from build123d import *

# Parameters (mm, degrees)
F0_W     = 330.2
F0_H     = 173.9225888619
F0_R     = 66.675
F1_DEPTH = 6.35


# Not quite as in the source:
# - the dataset's text gives a spline's control points without its knots; the knots are read off the source's solid


with BuildPart() as f1:
    # F0 (on Top) → F1 (new body)
    with BuildSketch(Plane.XY):
        with Locations((-132.4583572531, -73.9906652679)):
            Rectangle(F0_W, F0_H)
        with BuildLine():
            add(Edge.make_bspline(
                [(-138.9201402808, -141.3304854369), (-138.3928185407, -141.3304854369), (-137.3381750605, -141.275400301), (-135.2625215798, -140.9492902881), (-133.2552416123, -140.3064688013), (-131.3632448334, -139.3625418043), (-129.5649193209, -138.2239224731), (-127.5612000685, -136.4834555233), (-125.9244832491, -134.3798930655), (-124.862585277, -132.5093025607), (-123.9869219901, -130.5516065921), (-123.3950651292, -128.4884227829), (-123.095646983, -126.3629935264), (-123.0198869297, -124.7450926538), (-123.095646983, -123.1271917812), (-123.3950651292, -121.0017625246), (-123.9869219901, -118.9385787154), (-124.862585277, -116.9808827469), (-125.9244832491, -115.110292242), (-127.5612000685, -113.0067297843), (-129.5649193209, -111.2662628345), (-131.3632448334, -110.1276435032), (-133.2552416123, -109.1837165063), (-135.2625215798, -108.5408950195), (-137.3381750605, -108.2147850066), (-138.9201402808, -108.1321573027), (-140.5021055011, -108.2147850066), (-142.5777589818, -108.5408950195), (-144.5850389493, -109.1837165063), (-146.4770357282, -110.1276435032), (-148.2753612407, -111.2662628345), (-150.2790804931, -113.0067297843), (-151.9157973125, -115.110292242), (-152.9776952845, -116.9808827469), (-153.8533585715, -118.9385787154), (-154.4452154324, -121.0017625246), (-154.7446335786, -123.1271917812), (-154.8203936319, -124.7450926538), (-154.7446335786, -126.3629935264), (-154.4452154324, -128.4884227829), (-153.8533585715, -130.5516065921), (-152.9776952845, -132.5093025607), (-151.9157973125, -134.3798930655), (-150.2790804931, -136.4834555233), (-148.2753612407, -138.2239224731), (-146.4770357282, -139.3625418043), (-144.5850389493, -140.3064688013), (-142.5777589818, -140.9492902881), (-140.5021055011, -141.275400301), (-139.4474620209, -141.3304854369), (-138.9201402808, -141.3304854369)],
                knots=[0, 0, 0, 0, 0.015625, 0.03125, 0.0625, 0.078125, 0.09375, 0.125, 0.15625, 0.171875, 0.1875, 0.21875, 0.234375, 0.25, 0.265625, 0.28125, 0.3125, 0.328125, 0.34375, 0.375, 0.40625, 0.421875, 0.4375, 0.46875, 0.484375, 0.5, 0.515625, 0.53125, 0.5625, 0.578125, 0.59375, 0.625, 0.65625, 0.671875, 0.6875, 0.71875, 0.734375, 0.75, 0.765625, 0.78125, 0.8125, 0.828125, 0.84375, 0.875, 0.90625, 0.921875, 0.9375, 0.96875, 0.984375, 1, 1, 1, 1], degree=3))
        make_face(mode=Mode.SUBTRACT)
        with Locations((-219.2488735842, -58.1939341619)):
            Circle(F0_R, mode=Mode.SUBTRACT)
        with Locations((-45.6678409221, -58.1939341619)):
            Circle(F0_R, mode=Mode.SUBTRACT)
    extrude(amount=F1_DEPTH)


solid = f1.part
Model file for the job. Use its own axes, mm. Give positions to 0.01 mm unless a question says otherwise; leave off trailing zeros. Order: outer loops, then holes, each group sorted by start corner. A loop starts at its lowest first (then second) coordinate and runs counter-clockwise, first axis right, second up. Notation, with made-up numbers: M 12,-28.5 L 36,-28.5 A28 ccw 36,-9.5 Z; hole C 4,47.5 d5. An arc over 180 degrees is marked long. Put each result on its own line as item: value. Start each with the question number.
(1) Band-saw the part on B-B on y = -102. Give the cut face in (x, z).
(2) Pull direction Y, two halves, no side cores. Call faces 1 (the face through (-135, 12.971, 3)), 2 (the face through (17.93, -38.17, 3.13)), 3 (the face through (-135, -92, 0)): released by +Y, released by -Y, zero draft, split by the parting line, or undercut.
(3) Band-saw the part on A-A on x = -265. Give the cut face in (y, z), then the cut area to 3 significant figures.
(4) Band-saw the part on D-D on y = -26.5. Give the cut face in (x, z), then the cut area to 3 significant figures.
(5) Band-saw the part on C-C on x = -211.5. Give the cut face in (y, z).
(6) Drill centre lines: L1, parallel to Y at x = -218.5, z = 4.75; L2, parallel to X at y = -125, z = 2.5; L3, parallel to X at y = -83.5, z = 2.25. Where is each one in solid material? Low to high. Write a range as [from, to].
Results below:
1. outline: M -297.56,0 L -269.51,0 L -269.51,6.35 L -297.56,6.35 Z; M -168.98,0 L -95.93,0 L -95.93,6.35 L -168.98,6.35 Z; M 4.6,0 L 32.64,0 L 32.64,6.35 L 4.6,6.35 Z
2. face 1: released by +Y
2. face 2: undercut
2. face 3: zero draft
3. outline: M -160.95,0 L -106.7,0 L -106.7,6.35 L -160.95,6.35 Z; M -9.69,0 L 12.97,0 L 12.97,6.35 L -9.69,6.35 Z
3. area: 488 mm2
4. outline: M -297.56,0 L -277.91,0 L -277.91,6.35 L -297.56,6.35 Z; M -160.59,0 L -104.33,0 L -104.33,6.35 L -160.59,6.35 Z; M 12.99,0 L 32.64,0 L 32.64,6.35 L 12.99,6.35 Z
4. area: 607 mm2
5. outline: M -160.95,0 L -124.42,0 L -124.42,6.35 L -160.95,6.35 Z; M 8.03,0 L 12.97,0 L 12.97,6.35 L 8.03,6.35 Z
6. L1: y = [-160.95, -124.86], [8.48, 12.97]
6. L2: x = [-297.56, -154.79], [-123.05, 32.64]
6. L3: x = [-297.56, -280.93], [-157.56, -107.35], [16.02, 32.64]
